The figure shows three views and two pictorial views of one solid part (mm, origin at its lowest corner). Answer the questions. A direction names the side the tool comes from. Round coordinates to 2 decimals unless told otherwise and drop trailing zeros. Loops run counter-clockwise (first coordinate to the right, second up) from the corner with the lowest first, then second, coordinate; pieces in that order, holes last. Notation, with made-up numbers: (10, -36) -> (44, -36) arc R14 ccw to (44, -11) -> close; hole circle Ø6 at (37, 58). An arc over 180 degrees is marked (long way). Use a Markdown table: item, result. Add a question column.
Q1. Consider line 1 (X direction, y = 0.9, z = 4.15); line 2 (X direction, y = 3, z = 1.05) (3 decimals); line 3 (Y direction, x = 24.75, z = 4.05). Determine where each line is inside the solid, lowest interval first.
Q2. Section B-B on y = 1.9 is taken. Give the vertices of the cut face in (x, z), then the cut area to 3 significant figures.
Q3. Which of the six approach directions +Z, -Z, +X, -X, +Y, -Y give full straight-line access (tool end or side, diameter ignored) to the marked faces 1 and 2?
Q4. Section A-A on z = 2.8 is taken. Give the vertices of the cut face in (x, y), then the cut area to 3 significant figures.
Q5. Given pin 1 Ø3 at (y, z) = (3, 1) entering from -X; pin 2 Ø1 at (x, z) = (5.5, 3) entering from -Y; pin 3 Ø2.5 at (y, z) = (2.5, 3.5) entering from -X, each flat-ended and moving along its own axis, determine where each tip first touches the part or whether it passes through.
Q6. Section C-C on x = 24 is taken. Give the vertices of the cut face in (y, z), then the cut area to 3 significant figures.
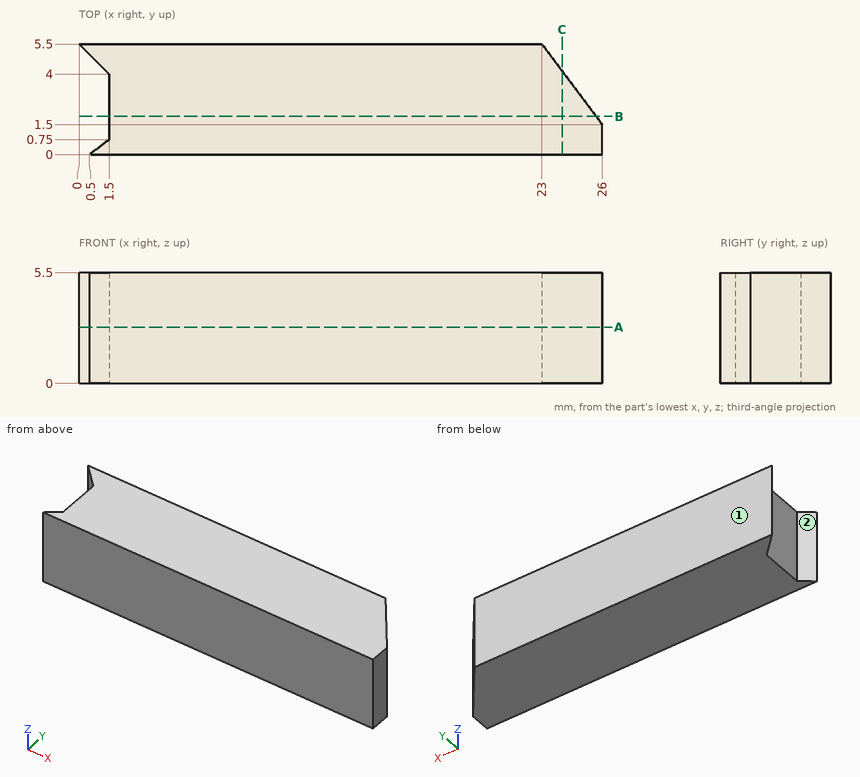
Checked values:
| question | item | result |
|---|---|---|
| 1 | line 1 | x = 1.5 to 26 |
| 1 | line 2 | x = 1.5 to 24.875 |
| 1 | line 3 | y = 0 to 3.17 |
| 2 | outline | (1.5, 0) -> (25.7, 0) -> (25.7, 5.5) -> (1.5, 5.5) -> close |
| 2 | area | 133 mm2 |
| 3 | face 1 | +Z, -Z, +X, -X, +Y |
| 3 | face 2 | +Z, -Z, -X |
| 4 | outline | (0, 5.5) -> (1.5, 4) -> (1.5, 0.75) -> (0.5, 0) -> (26, 0) -> (26, 1.5) -> (23, 5.5) -> close |
| 4 | area | 130 mm2 |
| 5 | pin 1 | stops at x = 1 |
| 5 | pin 2 | stops at y = 0 |
| 5 | pin 3 | stops at x = 1.5 |
| 6 | outline | (0, 0) -> (4.17, 0) -> (4.17, 5.5) -> (0, 5.5) -> close |
| 6 | area | 22.9 mm2 |
